Can you work these out from the model? Positions are in its coordinate system, mm. A direction names the side the tool comes from. Round coordinates to 2 decimals unless told otherwise and drop trailing zeros. Loops run counter-clockwise (first coordinate to the right, second up) from the corner with the lowest first, then second, coordinate; pieces in that order, holes last. Notation, with made-up numbers: M 21.5,69.25 L 52.5,69.25 A12 ccw 52.5,84.25 Z; hole C 71,-39.5 d6. An arc over 180 degrees is marked long. Use a Markdown table: item, result. Add a question column.
```python
from build123d import *

# Parameters (mm, degrees)
F0_W     = 121.92
F0_H     = 73.66
F1_DEPTH = 3.81
F2_R     = 16.556677
F3_R     = 8.202995
F3_R_2   = 5.144325
F3_R_3   = 4.381005
F3_R_4   = 5.718053
F4_DEPTH = 3.811


with BuildPart() as f1:
    # F0 (on Top) → F1 (new body)
    with BuildSketch(Plane.XY):
        with Locations((2.327671, 13.414853)):
            Rectangle(F0_W, F0_H)
    extrude(amount=F1_DEPTH)

    # F2
    f2_edges = [f1.edges().sort_by_distance(p)[0] for p in [
        (-58.632329, -23.415147, 1.905),
        (63.287671, -23.415147, 1.905),
        (63.287671, 50.244853, 1.905),
        (-58.632329, 50.244853, 1.905),
    ]]
    fillet(f2_edges, radius=F2_R)

    # F3 (on face) → F4 (cut, through all)
    with BuildSketch(Plane.XY.offset(3.81)):
        Polygon((-44.776369, 26.324741), (-34.277338, 31.26546), (-35.731862, 42.777398), (-47.129838, 44.951449), (-52.719651, 34.783147), align=None)
        Polygon((39.868699, 12.182859), (28.134486, 16.505987), (20.396876, 6.682008), (27.348982, -3.712673), (39.38323, -0.31296), align=None)
        Polygon((-39.143418, -7.019384), (-45.010525, -0.843484), (-52.697191, -4.514976), (-51.580704, -12.959983), (-43.204012, -14.507793), align=None)
        with Locations((-8.712908, 39.208088)):
            Circle(F3_R)
        with Locations((44.839598, -8.181633)):
            Circle(F3_R_2)
        with Locations((-24.438646, -15.831992)):
            Circle(F3_R_3)
        with Locations((52.277453, 41.970715)):
            Circle(F3_R_4)
        Polygon((-12.075472, 2.19376), (-25.326282, 15.444567), (-30.176412, -2.656374), align=None)
        Polygon((17.429908, 42.43333), (28.472248, 29.18253), (34.426607, 45.370877), align=None)
        Polygon((21.141237, -17.442858), (13.236605, -7.957305), (8.974191, -19.545694), align=None)
        Polygon((6.042457, 21.979525), (-0.092179, 19.034901), (-0.609377, 12.249838), (5.00806, 8.4094), (11.142695, 11.354025), (11.659894, 18.139087), align=None)
    extrude(amount=-F4_DEPTH, mode=Mode.SUBTRACT)


solid = f1.part
```
(1) Suppose I cut it at D-D on x = 3.5. List the corners of the cut face in (y, z) for me.
(2) Thinking about a two-plate mould opening in Y: for faces 1 (the face through (58.3, -18.7, 1.9)), 2 (the face through (-1.135, 36.066, 1.932)), 3 (the face through (2, 50.245, 2)), which applies, released by +Y, released by -Y, zero draft, split by the parting line, or undercut?
(3) Suppose I cut it at A-A on x = -37. List the corners of the cut face in (y, z) for me, and give its area (3 significant figures).
(4) Suppose I cut it at C-C on y = 14. List the corners of the cut face in (x, z) for me.
(5) Suppose I cut it at B-B on y = 4. List the corners of the cut face in (x, z) for me.
(6) If I drill on probe 1 along X at (y, z) = (3.5, 2.95); probe 2 along Y at (x, z) = (23.5, 0.65); probe 3 along X at (y, z) = (35.5, 2.7), over which ranges is the centre line in solid material (lowest first)? Write a range as [from, to].
(7) On a 3-axis mill with a long thin cutter (end or side, diameter ignored), from which of +Z, -Z, +X, -X, +Y, -Y can I reach the whole of each face in a straight line? I mean faces 4 (the face through (-27.717, 6.521, 1.932)), 5 (the face through (1, 6, 0)). Say none if no direction works.
Results below:
| question | item | result |
|---|---|---|
| 1 | outline | M -23.42,0 L 9.44,0 L 9.44,3.81 L -23.42,3.81 Z; M 20.76,0 L 50.24,0 L 50.24,3.81 L 20.76,3.81 Z |
| 2 | face 1 | released by -Y |
| 2 | face 2 | undercut |
| 2 | face 3 | released by +Y |
| 3 | outline | M -23.42,0 L 29.98,0 L 29.98,3.81 L -23.42,3.81 Z; M 43.02,0 L 50.24,0 L 50.24,3.81 L 43.02,3.81 Z |
| 3 | area | 231 mm² |
| 4 | outline | M -58.63,0 L -25.71,0 L -25.71,3.81 L -58.63,3.81 Z; M -23.88,0 L -0.48,0 L -0.48,3.81 L -23.88,3.81 Z; M 11.34,0 L 26.16,0 L 26.16,3.81 L 11.34,3.81 Z; M 34.94,0 L 63.29,0 L 63.29,3.81 L 34.94,3.81 Z |
| 5 | outline | M -58.63,0 L -28.39,0 L -28.39,3.81 L -58.63,3.81 Z; M -13.88,0 L 22.19,0 L 22.19,3.81 L -13.88,3.81 Z; M 39.55,0 L 63.29,0 L 63.29,3.81 L 39.55,3.81 Z |
| 6 | probe 1 | x = [-58.63, -28.53], [-13.38, 22.53], [39.53, 63.29] |
| 6 | probe 2 | y = [-23.42, 2.04], [10.62, 35.15], [43.48, 50.24] |
| 6 | probe 3 | x = [-58.53, -52.33], [-34.81, -16.03], [-1.4, 23.21], [30.8, 63.19] |
| 7 | face 4 | +Z, -Z |
| 7 | face 5 | -Z, +X, -X, +Y, -Y |
